from build123d import *

# Parameters (mm, degrees)
SKETCH1_R           = 22.5
BOSS_EXTRUDE1_DEPTH = 20
SKETCH2_R           = 10
CUT_EXTRUDE1_DEPTH  = 20
SKETCH3_R           = 1.5
CUT_EXTRUDE2_DEPTH  = 20
SKETCH4_R           = 21
CUT_EXTRUDE3_DEPTH  = 18


with BuildPart() as part:
    # Sketch1 → Boss-Extrude1 (new body)
    with BuildSketch(Plane.XY):
        Circle(SKETCH1_R)
        with BuildLine():
            Line((-17.123625514, -14.595596913), (-17.123625514, -76.9))
            Line((-17.123625514, -76.9), (16.876374486, -76.9))
            Line((16.876374486, -76.9), (16.876374486, -14.880792459))
            ThreePointArc((16.876374486, -14.880792459), (-0.188725707, -22.499208488), (-17.123625514, -14.595596913))
        make_face()
    extrude(amount=BOSS_EXTRUDE1_DEPTH)

    # Sketch2 → Cut-Extrude1 (cut)
    with BuildSketch(Plane(origin=(0, 0, 0), x_dir=(-1, 0, 0), z_dir=(0, 0, -1))):
        Circle(SKETCH2_R)
    extrude(amount=-CUT_EXTRUDE1_DEPTH, mode=Mode.SUBTRACT)

    # Sketch3 → Cut-Extrude2 (cut)
    with BuildSketch(Plane(origin=(0, 0, 0), x_dir=(-1, 0, 0), z_dir=(0, 0, -1))):
        with Locations((0, 15)):
            Circle(SKETCH3_R)
        with Locations((12.990381057, -7.5)):
            Circle(SKETCH3_R)
        with Locations((-12.990381057, -7.5)):
            Circle(SKETCH3_R)
    extrude(amount=-CUT_EXTRUDE2_DEPTH, mode=Mode.SUBTRACT)

    # Sketch4 → Cut-Extrude3 (cut)
    with BuildSketch(Plane(origin=(0, 0, 0), x_dir=(-1, 0, 0), z_dir=(0, 0, -1))):
        Circle(SKETCH4_R)
    extrude(amount=-CUT_EXTRUDE3_DEPTH, mode=Mode.SUBTRACT)


solid = part.part
Can you work these out from the model? Positions are in its coordinate system, mm. A direction names the side the tool comes from. Coordinates: 2 decimals unless noted, no trailing zeros. Write each loop counter-clockwise with the first axis right and the second up, starting at its lowest first coordinate (ties: lowest second). Pieces come first, ordered by that corner, then holes. Notation, with made-up numbers: (30.25, 31.5) -> (86.25, 31.5) arc R24 cw to (86.25, 51.5) -> close; hole circle Ø3 at (28.5, 26). An arc over 180 degrees is marked (long way). Write each question's results on one line, items separated by ' | '. Start each with the question number.
Item 1: If we section it at C-C, the plane z = 7.25: Write out the boundary of the cut face in (x, y), and give its area (3 significant figures).
Item 2: On a 3-axis mill with a long thin cutter (end or side, diameter ignored), from which of +Z, -Z, +X, -X, +Y, -Y can I reach the whole of each face in a straight line? I mean faces 4 (the flat face through (0, -76.9, 10)), 5 (the flat face through (-17.124, -45, 10)), 6 (the cylindrical face through (-20.03, 6.31, 8.87)). Say none if no direction works.
Item 3: I'm going to push flat-ended pins straight in: P1, Ø10, axis at y = -50.5, z = 17, coming from the +X side; P2, Ø2, axis at y = 12.5, z = 17.5, coming from the +X side; P3, Ø5, axis at y = -3, z = 17, coming from the +X side; P4, Ø2.5, axis at x = -12.99, y = -7.5, coming from the +Z side. Where does each tip first touch, or does it pass through?
Item 4: If we section it at B-B, the plane y = 0: Write out the boundary of the cut face in (x, z), and give its area (3 significant figures).
Item 5: If we section it at D-D, the plane x = 12.5: Write out the boundary of the cut face in (y, z), and give its area (3 significant figures).
Item 6: Thinking about a two-plate mould opening in Y: for faces 1 (the flat face through (16.876, -46, 10)), 2 (the cylindrical face through (0.91, 22.48, 9.86)), 3 (the cylindrical face through (-13.68, -8.83, 18.99)), which applies, released by +Y, released by -Y, zero draft, split by the parting line, or undercut?
Item 7: Please list where these lines run through material, in increasing order: probe 1 along Y at (x, z) = (0, 18.4); probe 2 along Y at (x, z) = (0, 13.75); probe 3 along Z at (x, y) = (-1, -15.5).
Item 8: If we section it at A-A, the plane x = 0: Write out the boundary of the cut face in (y, z).
Answer block:
1) outline: (-17.12, -76.9) -> (16.88, -76.9) -> (16.88, -14.88) arc R22.5 ccw (long way) to (-17.12, -14.6) -> close; hole circle Ø42 at (0, 0) | area: 2,140 mm²
2) face 4: +Z, -Z, +X, -X, -Y | face 5: +Z, -Z, -X, -Y | face 6: -Z
3) P1: x = 16.88 | P2: x = 19.34 | P3: x = 22.49 | P4: through
4) outline: (-22.5, 0) -> (-21, 0) -> (-21, 18) -> (-10, 18) -> (-10, 20) -> (-22.5, 20) -> close; (10, 18) -> (21, 18) -> (21, 0) -> (22.5, 0) -> (22.5, 20) -> (10, 20) -> close | area: 104 mm²
5) outline: (-76.9, 0) -> (-16.87, 0) -> (-16.87, 18) -> (-8.92, 18) -> (-8.92, 20) -> (-76.9, 20) -> close; (-6.08, 18) -> (16.87, 18) -> (16.87, 0) -> (18.71, 0) -> (18.71, 20) -> (-6.08, 20) -> close | area: 1,300 mm²
6) face 1: zero draft | face 2: split by the parting line | face 3: undercut
7) probe 1: -76.9 to -10, 10 to 13.5, 16.5 to 22.5 | probe 2: -76.9 to -21, 21 to 22.5 | probe 3: 18 to 20
8) outline: (-76.9, 0) -> (-21, 0) -> (-21, 18) -> (-10, 18) -> (-10, 20) -> (-76.9, 20) -> close; (10, 18) -> (13.5, 18) -> (13.5, 20) -> (10, 20) -> close; (16.5, 18) -> (21, 18) -> (21, 0) -> (22.5, 0) -> (22.5, 20) -> (16.5, 20) -> close
